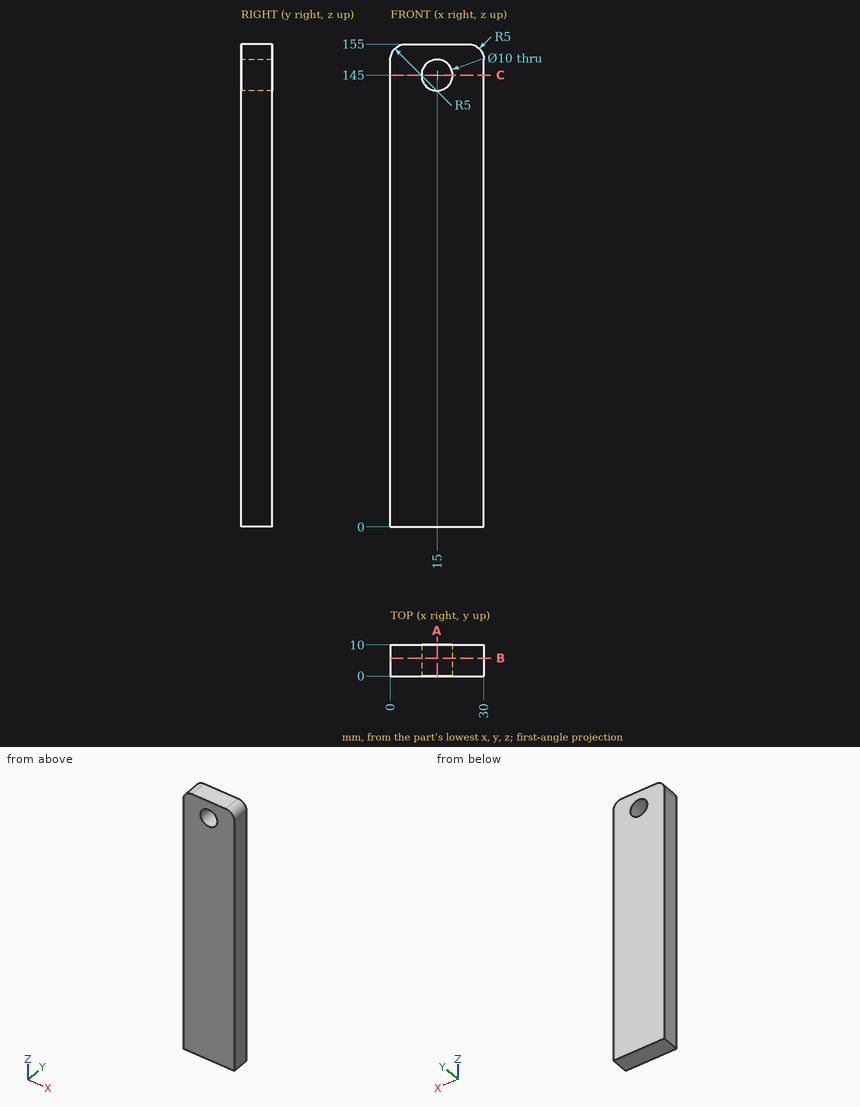
Drawing for the job (mm, zero at the part's lowest x, y, z). Round coordinates to 2 decimals unless told otherwise and drop trailing zeros. Loops run counter-clockwise (first coordinate to the right, second up) from the corner with the lowest first, then second, coordinate; pieces in that order, holes last.
1. Wall check: probe 1 along X at (y, z) = (5.5, 145); probe 2 along Z at (x, y) = (14.5, 0.5); probe 3 along X at (y, z) = (0.75, 143.5). Give the ranges that are in metal, low to high.
Check values:
probe 1: x = 0 to 10, 20 to 30
probe 2: z = 0 to 140.03, 149.97 to 155
probe 3: x = 0 to 10.23, 19.77 to 30
2. Band-saw the part on A-A, the plane x = 15. List the corners of the cut face in (y, z).
Check values:
outline: (0, 0) - (10, 0) - (10, 140) - (0, 140) - close; (0, 150) - (10, 150) - (10, 155) - (0, 155) - close
3. Band-saw the part on C-C, the plane z = 145. List the corners of the cut face in (x, y).
Check values:
outline: (0, 0) - (10, 0) - (10, 10) - (0, 10) - close; (20, 0) - (30, 0) - (30, 10) - (20, 10) - close
4. Band-saw the part on B-B, the plane y = 5.75. List the corners of the cut face in (x, z), and give its area (3 significant figures).
Check values:
outline: (0, 0) - (30, 0) - (30, 150) arc R5 ccw to (25, 155) - (5, 155) arc R5 ccw to (0, 150) - close; hole circle Ø10 at (15, 145)
area: 4,560 mm2
5. Drop a flat-ended pin along its axis: P1, Ø6, axis at x = 15, z = 145, coming from the +Y side. Give the stop position or say it passes through.
Check values:
P1: passes through
